Autodesk Inventor part; units mm, degrees
ref_plane "YZ Plane" through (0, 0, 0) normal (1, 0, 0) x (0, 1, 0)
ref_plane "XZ Plane" through (0, 0, 0) normal (0, 1, 0) x (-1, 0, 0)
ref_plane "XY Plane" through (0, 0, 0) normal (0, 0, 1) x (1, 0, 0)
sketch "Эскиз1" plane through (0, 0, 0) normal (0, 0, 1) x (1, 0, 0)
  line L0 (-4.7, 2.25) -> (4.7, 2.25)
  line L1 (4.7, 2.25) -> (4.7, -2.25)
  line L2 (4.7, -2.25) -> (-4.7, -2.25)
  line L3 (-4.7, -2.25) -> (-4.7, 2.25)
  point P0 (0, 0)
  point P1 (-4.7, 0)
  point P2 (0, 2.25)
  dimension "d0" = 9.4
  dimension "d1" = 4.5
extrude "Выдавливание1" add sketch "Эскиз1" along normal mid plane 10.2
sketch "Эскиз3" plane through (0, 0, 5.1) normal (0, 0, 1) x (1, 0, 0)
  line L0 (-4.7, 2.25) -> (-4.7, -2.25)
  line L1 (-4.7, 0.75) -> (-2.9, 0.75)
  line L2 (-2.9, 0.75) -> (-2.9, 2.25)
  line L3 (4.7, 2.25) -> (-4.7, 2.25)
  line L4 (4.7, -2.25) -> (4.7, 2.25)
  line L5 (4.7, 0.75) -> (2.9, 0.75)
  line L6 (2.9, 0.75) -> (2.9, 2.25)
  point P0 (0, 0)
  dimension "d7" = 1.5
  dimension "d8" = 2.9
  dimension "d9" = 5.8
extrude "Выдавливание2" cut sketch "Эскиз3" against normal blind 10.2
sketch "Эскиз5" plane through (0, 0, 5.1) normal (0, 0, 1) x (1, 0, 0)
  line L0 (-4.7, -2.25) -> (4.7, -2.25)
  line L1 (-2.9, -2.25) -> (-4.7, -0.75)
  line L2 (-4.7, 0.75) -> (-4.7, -2.25)
  line L3 (4.7, -2.25) -> (4.7, 0.75)
  line L4 (4.7, -0.75) -> (2.9, -2.25)
  point P0 (0, 0)
  dimension "d15" = 1.5
  dimension "d16" = 2.9
  dimension "d17" = 5.8
extrude "Выдавливание3" cut sketch "Эскиз5" against normal blind 10.2
sketch "Эскиз6" plane through (-2.9, 2.25, -5.1) normal (0, 1, 0) x (1, 0, 0)
  point P0 (2.9, -5.1)
  point P1 (2.9, -5.1)
hole "Отверстие1" at (0, 2.25, 0) direction (0, -1, 0) diameter 4 end through all
thread "Резьба1"
chamfer "Фаска1" distance 0.2 angle 45 2 edges at (0, 2.25, -2) (0, -2.25, -2)
fillet "Сопряжение2" radius 0.1 2 edges at (2.9, 2.25, 0) (-2.9, 2.25, 0)
fillet "Сопряжение3" radius 0.3 2 edges at (-4.7, 0.75, 0) (4.7, 0.75, 0)
properties part number "COTS_GENERIC_20x20_M4_Nut" material "Сталь"
Geometry check sheet. Reference: the model listing, model coordinates, mm. A direction names the side the tool comes from. Give positions to 0.01 mm unless a question says otherwise; leave off trailing zeros. Order: outer loops, then holes, each group sorted by start corner. A loop starts at its lowest first (then second) coordinate and runs counter-clockwise, first axis right, second up. Notation, with made-up numbers: (19, -3.75) - (78, -3.75) arc R19 cw to (78, 0.25) - close; hole circle Ø9 at (52.25, -8). An arc over 180 degrees is marked (long way). Answer as a JSON object with one key per item and string values.
(1) Material ranges on line 1 (Z direction, x = 0, y = -1.15); line 2 (X direction, y = -0.5, z = 0); line 3 (X direction, y = -1, z = 2.25), recorded low to high.
Report:
{"line 1": "-5.1 to -2, 2 to 5.1", "line 2": "-4.7 to -2, 2 to 4.7", "line 3": "-4.4 to 4.4"}
(2) Cross-section at B-B (x = 0). Record the cut outline in (y, z).
Report:
{"outline": "(-2.25, -5.1) - (2.25, -5.1) - (2.25, -2.2) - (2.05, -2) - (-2.05, -2) - (-2.25, -2.2) - close; (-2.25, 2.2) - (-2.05, 2) - (2.05, 2) - (2.25, 2.2) - (2.25, 5.1) - (-2.25, 5.1) - close"}
(3) Cross-section at A-A (z = 0). Record the cut outline in (x, y).
Report:
{"outline": "(-4.7, -0.75) - (-2.9, -2.25) - (-2.2, -2.25) - (-2, -2.05) - (-2, 2.05) - (-2.2, 2.25) - (-2.8, 2.25) arc R0.1 ccw to (-2.9, 2.15) - (-2.9, 0.75) - (-4.4, 0.75) arc R0.3 ccw to (-4.7, 0.45) - close; (2, -2.05) - (2.2, -2.25) - (2.9, -2.25) - (4.7, -0.75) - (4.7, 0.45) arc R0.3 ccw to (4.4, 0.75) - (2.9, 0.75) - (2.9, 2.15) arc R0.1 ccw to (2.8, 2.25) - (2.2, 2.25) - (2, 2.05) - close"}
(4) Cross-section at C-C (y = 1.3). Record the cut outline in (x, z), then the cut area to 3 significant figures.
Report:
{"outline": "(-2.9, -5.1) - (2.9, -5.1) - (2.9, 5.1) - (-2.9, 5.1) - close; hole circle Ø4 at (0, 0)", "area": "46.6 mm^2"}
(5) Cross-section at D-D (y = -1.25). Record the cut outline in (x, z), then the cut area to 3 significant figures.
Report:
{"outline": "(-4.1, -5.1) - (4.1, -5.1) - (4.1, 5.1) - (-4.1, 5.1) - close; hole circle Ø4 at (0, 0)", "area": "71.1 mm^2"}
(6) Depth check by flat-ended pin: pin 1 Ø1.7 at (x, z) = (-3.5, 2) entering from +Y; pin 2 Ø1.1 at (y, z) = (1.5, -1.5) entering from +X; pin 3 Ø0.8 at (x, z) = (3.5, 2) entering from +Y; pin 4 Ø2.5 at (x, z) = (0, 0) entering from +Y. Enter the tip coordinate at first touch or a pass-through.
Report:
{"pin 1": "y = 2.25", "pin 2": "x = 2.9", "pin 3": "y = 0.75", "pin 4": "through"}
(7) Draft check along Z on faces 1 (the cylindrical face through (2, 0, 0)), 2 (the flat face through (0, 0, 5.1)), 3 (the flat face through (0, 0, -5.1)), 4 (the flat face through (2.9, 1, 0)). Enter one of: released by +Z, released by -Z, zero draft, split by the parting line, or undercut.
Report:
{"face 1": "undercut", "face 2": "released by +Z", "face 3": "released by -Z", "face 4": "zero draft"}
(8) Tool access check on faces 5 (the flat face through (4, 0.75, 0)), 6 (the flat face through (-2.9, 1, 0)), 7 (the flat face through (-4.7, 0, 0)). Record the directions out of +Z, -Z, +X, -X, +Y, -Y that give a thin tool (end or side, any length) a straight path to the whole face; none if there is none.
Report:
{"face 5": "+Z, -Z, +X, +Y", "face 6": "+Z, -Z, -X, +Y", "face 7": "+Z, -Z, -X, +Y, -Y"}
